```python
from build123d import *

# Parameters (mm, degrees)
SKETCH1_R           = 7.5
SKETCH1_R_2         = 4.7
SKETCH1_R_3         = 2.1
BOSS_EXTRUDE1_DEPTH = 4
BOSS_EXTRUDE2_START = 4
SKETCH1_3_R         = 4.7
SKETCH1_3_R_2       = 2.1
BOSS_EXTRUDE2_DEPTH = 26
CUT_EXTRUDE1_START  = 30
SKETCH1_4_R         = 2.1
CUT_EXTRUDE1_DEPTH  = 10
FILLET1_R           = 1.5


with BuildPart() as part:
    # Sketch1 → Boss-Extrude1 (new body)
    with BuildSketch(Plane(origin=(0, 0, 0), x_dir=(1, 0, 0), z_dir=(0, 1, 0))):
        with Locations(Location((0, 0, 0), (0, 0, 270))):
            Circle(SKETCH1_R)
        Circle(SKETCH1_R_2, mode=Mode.SUBTRACT)
        Circle(SKETCH1_R_2)
        Circle(SKETCH1_R_3, mode=Mode.SUBTRACT)
        Circle(SKETCH1_R_3)
    extrude(amount=BOSS_EXTRUDE1_DEPTH)

    # Sketch1<3> → Boss-Extrude2 (add)
    with BuildSketch(Plane(origin=(0, 0, 0), x_dir=(1, 0, 0), z_dir=(0, 1, 0)).offset(BOSS_EXTRUDE2_START)):
        with Locations(Location((0, 0, 0), (0, 0, 90))):
            Circle(SKETCH1_3_R)
        Circle(SKETCH1_3_R_2, mode=Mode.SUBTRACT)
        Circle(SKETCH1_3_R_2)
    extrude(amount=BOSS_EXTRUDE2_DEPTH)

    # Sketch1<4> → Cut-Extrude1 (cut)
    with BuildSketch(Plane(origin=(0, 0, 0), x_dir=(1, 0, 0), z_dir=(0, 1, 0)).offset(CUT_EXTRUDE1_START)):
        with Locations(Location((0, 0, 0), (0, 0, 270))):
            Circle(SKETCH1_4_R)
    extrude(amount=-CUT_EXTRUDE1_DEPTH, mode=Mode.SUBTRACT)

    # Fillet1
    fillet1_edges = [part.edges().sort_by_distance(p)[0] for p in [
        (0, 4, 4.7),
    ]]
    fillet(fillet1_edges, radius=FILLET1_R)


solid = part.part
```
Geometry: final body of the model. Coordinates: model frame, mm. A direction names the side the tool comes from. Coordinates: 2 decimals unless noted, no trailing zeros. Order: outer loops, then holes, each group sorted by start corner. A loop starts at its lowest first (then second) coordinate and runs counter-clockwise, first axis right, second up. Notation, with made-up numbers: (16.5, 13) -> (37.5, 13) arc R13 cw to (37.5, 31) -> close; hole circle Ø6 at (-35, 47.5). An arc over 180 degrees is marked (long way). Answer in a Markdown table with one row per item.
Item 1: Draft query along X for faces 1 (the flat face through (0, 0, 0)), 2 (the cylindrical face through (-1.412, 17.578, -4.483)), 3 (the cylindrical face through (0.631, 25.07, 2.003)). Return one class per face: released by +X, released by -X, zero draft, split by the parting line, or undercut.
Return value:
| item | result |
|---|---|
| face 1 | zero draft |
| face 2 | split by the parting line |
| face 3 | undercut |
Item 2: Section D-D on y = 15. Output: boundary loops of the cut face in (x, z), plus the area to 3 significant figures.
Return value:
| item | result |
|---|---|
| outline | circle Ø9.4 at (0, 0) |
| area | 69.4 mm² |
Item 3: Ray query, L1, parallel to X at y = 27, z = 0; L2, parallel to Y at x = -6.5, z = 2; L3, parallel to Z at x = 0.25, y = 15.5. Return the intervals inside material, ascending.
Return value:
| item | result |
|---|---|
| L1 | x = -4.7 to -2.1, 2.1 to 4.7 |
| L2 | y = 0 to 4 |
| L3 | z = -4.69 to 4.69 |
Item 4: Access query for faces 4 (the flat face through (6, 4, -3)), 5 (the cylindrical face through (0.33, 1.972, -7.493)). Directions: +Z, -Z, +X, -X, +Y, -Y. A direction counts if a zero-diameter tool reaches every point of the face in a straight line with its end or side. Return the directions, or none.
Return value:
| item | result |
|---|---|
| face 4 | +Y |
| face 5 | +Y, -Y |
Item 5: Section B-B on x = 0. Output: boundary loops of the cut face in (y, z), plus the area to 3 significant figures.
Return value:
| item | result |
|---|---|
| outline | (0, -7.5) -> (4, -7.5) -> (4, -6.2) arc R1.5 cw to (5.5, -4.7) -> (30, -4.7) -> (30, -2.1) -> (20, -2.1) -> (20, 2.1) -> (30, 2.1) -> (30, 4.7) -> (5.5, 4.7) arc R1.5 cw to (4, 6.2) -> (4, 7.5) -> (0, 7.5) -> close |
| area | 263 mm² |
Item 6: Contact query for flat-ended pins moving along their axis: P1, Ø5, axis at x = -2, y = 11.5, coming from the +Z side; P2, Ø3, axis at x = -5, y = 17.5, coming from the -Z side; P3, Ø6, axis at x = 3, y = 5, coming from the +Z side. Output: stop coordinate, or through.
Return value:
| item | result |
|---|---|
| P1 | stops at z = 4.7 |
| P2 | stops at z = -3.14 |
| P3 | stops at z = 7.5 |
Item 7: Section C-C on y = 27.25. Output: boundary loops of the cut face in (x, z).
Return value:
| item | result |
|---|---|
| outline | circle Ø9.4 at (0, 0); hole circle Ø4.2 at (0, 0) |
Item 8: Section A-A on z = 0. Output: boundary loops of the cut face in (x, y).
Return value:
| item | result |
|---|---|
| outline | (-7.5, 0) -> (7.5, 0) -> (7.5, 4) -> (6.2, 4) arc R1.5 cw to (4.7, 5.5) -> (4.7, 30) -> (2.1, 30) -> (2.1, 20) -> (-2.1, 20) -> (-2.1, 30) -> (-4.7, 30) -> (-4.7, 5.5) arc R1.5 cw to (-6.2, 4) -> (-7.5, 4) -> close |
